Geometry check sheet. Reference: the model listing, model coordinates, mm. A direction names the side the tool comes from. Give positions to 0.01 mm unless a question says otherwise; leave off trailing zeros. Write each loop counter-clockwise with the first axis right and the second up, starting at its lowest first coordinate (ties: lowest second). Pieces come first, ordered by that corner, then holes. Notation, with made-up numbers: (-17, -7) -> (28, -7) arc R29 ccw to (28, 16) -> close; hole circle Ø8 at (19.25, -28.75). An arc over 180 degrees is marked (long way). Use a Markdown table: item, result. Add a question column.
from build123d import *

# Parameters (mm, degrees)
SKETCH_1_R          = 8.5
EXTRUDE_1_DEPTH     = 7
SKETCH_3_R          = 14
CUT_EXTRUDE_2_DEPTH = 5
CUT_EXTRUDE_3_REACH = 119.389
SKETCH_4_R          = 2.5
CUT_EXTRUDE_5_REACH = 119.389
SKETCH_6_W          = 53
SKETCH_6_H          = 15
EXTRUDE_START       = -7
EXTRUDE_2_DEPTH     = 7


with BuildPart() as part:
    # 草图1 → 凸台-拉伸1 (new body)
    with BuildSketch(Plane.XY):
        with BuildLine():
            ThreePointArc((20.155644371, 10), (0, 22.5), (-20.155644371, 10))
            Line((-20.155644371, 10), (-105, 10))
            ThreePointArc((-105, 10), (-115, 0), (-105, -10))
            Line((-105, -10), (-20.155644371, -10))
            ThreePointArc((-20.155644371, -10), (0, -22.5), (20.155644371, -10))
            Line((20.155644371, -10), (105, -10))
            ThreePointArc((105, -10), (115, 0), (105, 10))
            Line((105, 10), (20.155644371, 10))
        make_face()
        Circle(SKETCH_1_R, mode=Mode.SUBTRACT)
    extrude(amount=-EXTRUDE_1_DEPTH)

    # 草图3 → 切除-拉伸2 (cut)
    with BuildSketch(Plane(origin=(0, 0, -7), x_dir=(-1, 0, 0), z_dir=(0, 0, -1))):
        Circle(SKETCH_3_R)
    extrude(amount=-CUT_EXTRUDE_2_DEPTH, mode=Mode.SUBTRACT)

    # 草图4 → 切除-拉伸3 (cut, up to next)
    with BuildSketch(Plane.XY.offset(-7), mode=Mode.PRIVATE) as cut_extrude_3_sk1:
        with Locations((30, 0)):
            Circle(SKETCH_4_R)
    cut_extrude_3_tool1 = extrude(cut_extrude_3_sk1.sketch, amount=CUT_EXTRUDE_3_REACH, mode=Mode.PRIVATE) & part.part
    # 草图4 → 切除-拉伸3 (cut, up to next)
    with BuildSketch(Plane.XY.offset(-7), mode=Mode.PRIVATE) as cut_extrude_3_sk2:
        with Locations((105, 0)):
            Circle(SKETCH_4_R)
    cut_extrude_3_tool2 = extrude(cut_extrude_3_sk2.sketch, amount=CUT_EXTRUDE_3_REACH, mode=Mode.PRIVATE) & part.part
    # 草图4 → 切除-拉伸3 (cut, up to next)
    with BuildSketch(Plane.XY.offset(-7), mode=Mode.PRIVATE) as cut_extrude_3_sk3:
        with Locations(Location((-105, 0, 0), (0, 0, 180))):
            Circle(SKETCH_4_R)
    cut_extrude_3_tool3 = extrude(cut_extrude_3_sk3.sketch, amount=CUT_EXTRUDE_3_REACH, mode=Mode.PRIVATE) & part.part
    # 草图4 → 切除-拉伸3 (cut, up to next)
    with BuildSketch(Plane.XY.offset(-7), mode=Mode.PRIVATE) as cut_extrude_3_sk4:
        with Locations(Location((-30, 0, 0), (0, 0, 180))):
            Circle(SKETCH_4_R)
    cut_extrude_3_tool4 = extrude(cut_extrude_3_sk4.sketch, amount=CUT_EXTRUDE_3_REACH, mode=Mode.PRIVATE) & part.part
    add(cut_extrude_3_tool1.solids().sort_by_distance((30, 0, -7))[0], mode=Mode.SUBTRACT)
    add(cut_extrude_3_tool2.solids().sort_by_distance((105, 0, -7))[0], mode=Mode.SUBTRACT)
    add(cut_extrude_3_tool3.solids().sort_by_distance((-105, 0, -7))[0], mode=Mode.SUBTRACT)
    add(cut_extrude_3_tool4.solids().sort_by_distance((-30, 0, -7))[0], mode=Mode.SUBTRACT)

    # 草图6 → 切除-拉伸5 (cut, up to next)
    with BuildSketch(Plane(origin=(0, 0, -7), x_dir=(-1, 0, 0), z_dir=(0, 0, -1)), mode=Mode.PRIVATE) as cut_extrude_5_sk1:
        with Locations((-67.5, 2.5)):
            Rectangle(SKETCH_6_W, SKETCH_6_H)
    cut_extrude_5_tool1 = extrude(cut_extrude_5_sk1.sketch, amount=-CUT_EXTRUDE_5_REACH, mode=Mode.PRIVATE) & part.part
    # 草图6 → 切除-拉伸5 (cut, up to next)
    with BuildSketch(Plane(origin=(0, 0, -7), x_dir=(-1, 0, 0), z_dir=(0, 0, -1)), mode=Mode.PRIVATE) as cut_extrude_5_sk2:
        with Locations((67.5, 2.5)):
            Rectangle(SKETCH_6_W, SKETCH_6_H)
    cut_extrude_5_tool2 = extrude(cut_extrude_5_sk2.sketch, amount=-CUT_EXTRUDE_5_REACH, mode=Mode.PRIVATE) & part.part
    add(cut_extrude_5_tool1.solids().sort_by_distance((67.5, 2.5, -7))[0], mode=Mode.SUBTRACT)
    add(cut_extrude_5_tool2.solids().sort_by_distance((-67.5, 2.5, -7))[0], mode=Mode.SUBTRACT)

    # 草图7 → 凸台-拉伸2 (add)
    with BuildSketch(Plane(origin=(0, 0, -7), x_dir=(-1, 0, 0), z_dir=(0, 0, -1)).offset(EXTRUDE_START)):
        with BuildLine():
            ThreePointArc((-105, -10), (-52.870714977, -19.364005631), (-4.1e-08, -22.5))
            ThreePointArc((-4.1e-08, -22.5), (-11.858541243, -19.121323165), (-20.155644371, -10))
            Line((-20.155644371, -10), (-105, -10))
        make_face()
        with BuildLine():
            Line((105, -10), (20.155644371, -10))
            ThreePointArc((20.155644371, -10), (11.858541208, -19.121323187), (-4.1e-08, -22.5))
            ThreePointArc((-4.1e-08, -22.5), (52.870714936, -19.364005636), (105, -10))
        make_face()
    extrude(amount=EXTRUDE_2_DEPTH)


solid = part.part
1) Sectioned sample at C-C, the plane x = -30. Enter the section's corners in (y, z).
2) Tool access check on faces 4 (the face through (4.57, 7.167, -0.986)), 5 (the face through (-12.932, -5.362, -4.535)), 6 (the face through (-30, 10, -3)), 7 (the face through (100, 10, -3)), 8 (the face through (-94, 2, -4)). Record the directions out of +Z, -Z, +X, -X, +Y, -Y that give a thin tool (end or side, any length) a straight path to the whole face; none if there is none.
3) Sectioned sample at A-A, the plane z = -3.5. Enter the section's corners in (x, y).
4) Sectioned sample at B-B, the plane y = 0. Count the separate pieces of the cut face and the enclosed holes in it, and give its area (3 significant figures).
5) Gauge pin test, flat ends, axial feed: P1, Ø12, axis at x = -20, y = 3.5, coming from the +Z side; P2, Ø2, axis at x = 101.5, z = -4.5, coming from the +Y side; P3, Ø4.5, axis at x = 105, y = 0, coming from the +Z side. Record the tip position at first contact, or that the pin passes through.
6) Material ranges on probe 1 along Y at (x, z) = (-105, -1.5); probe 2 along Z at (x, y) = (1, 10.5); probe 3 along Y at (x, z) = (88.5, -2.25), recorded low to high. Write a range as [from, to].
7) Sectioned sample at D-D, the plane y = -12. Enter the section's corners in (x, z), and give its area (3 significant figures).
8) Draft check along X on faces 1 (the face through (-99, 10, -3)), 2 (the face through (-67, -5, -4)), 3 (the face through (0.3, 22.5, -3.5)). Enter one of: +X half, -X half, draft (parallel to the pull), parting line (faces both ways), or undercut.
Check values:
| question | item | result |
|---|---|---|
| 1 | outline | (-21.49, -7) -> (-2.5, -7) -> (-2.5, 0) -> (-21.49, 0) -> close; (2.5, -7) -> (10, -7) -> (10, 0) -> (2.5, 0) -> close |
| 2 | face 4 | +Z, -Z |
| 2 | face 5 | -Z |
| 2 | face 6 | +Z, -Z, -X, +Y |
| 2 | face 7 | +Z, -Z, +X, +Y |
| 2 | face 8 | +Z, -Z, +Y |
| 3 | outline | (-105, -10) arc R447.25 ccw to (105, -10) arc R10 ccw to (105, 10) -> (94, 10) -> (94, -5) -> (41, -5) -> (41, 10) -> (20.16, 10) arc R22.5 ccw to (-20.16, 10) -> (-41, 10) -> (-41, -5) -> (-94, -5) -> (-94, 10) -> (-105, 10) arc R10 ccw to start; hole circle Ø5 at (-105, 0); hole circle Ø5 at (-30, 0); hole circle Ø28 at (0, 0); hole circle Ø5 at (30, 0); hole circle Ø5 at (105, 0) |
| 4 | separate pieces | 8 |
| 4 | enclosed holes | 0 |
| 4 | area | 554 mm² |
| 5 | P1 | z = 0 |
| 5 | P2 | y = 10 |
| 5 | P3 | through |
| 6 | probe 1 | [-10, -2.5], [2.5, 10] |
| 6 | probe 2 | [-2, 0] |
| 6 | probe 3 | [-13.66, -5] |
| 7 | outline | (-96.34, -7) -> (-7.21, -7) -> (-7.21, -2) -> (7.21, -2) -> (7.21, -7) -> (96.34, -7) -> (96.34, 0) -> (-96.34, 0) -> close |
| 7 | area | 1,280 mm² |
| 8 | face 1 | draft |
| 8 | face 2 | undercut |
| 8 | face 3 | parting line |
